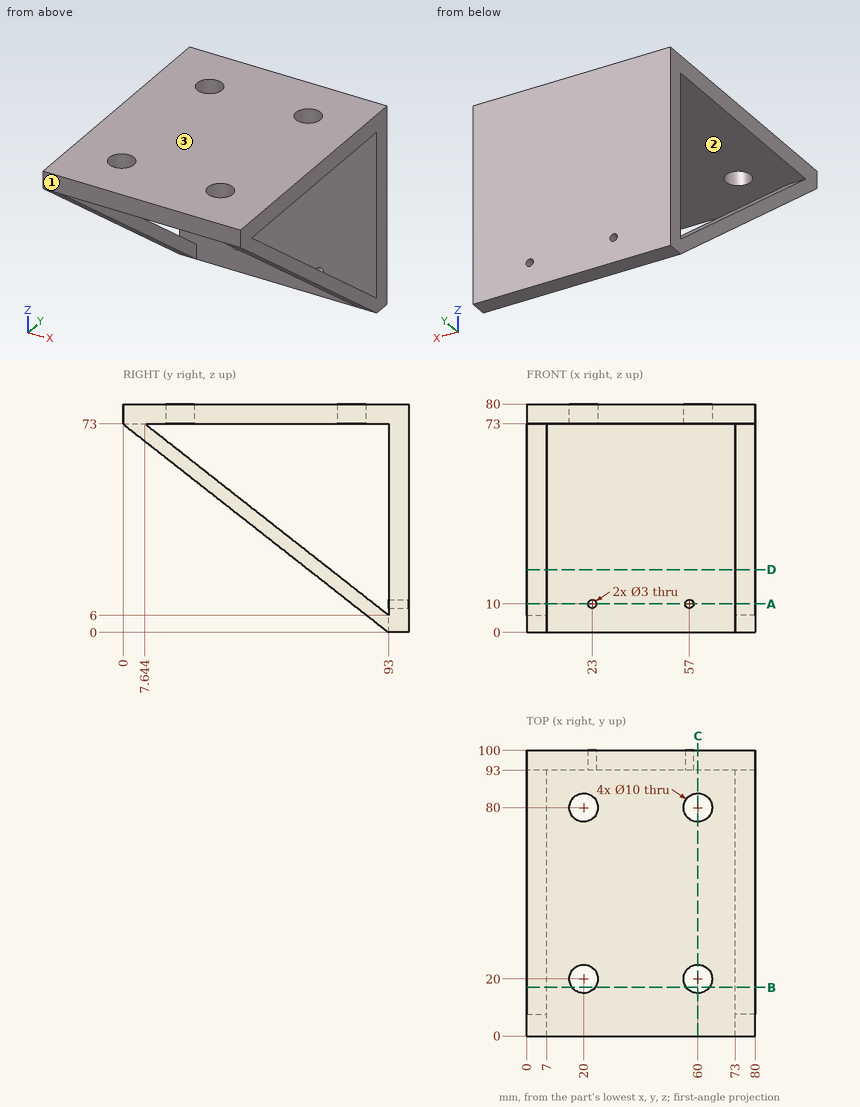
The figure shows three views and two pictorial views of one solid part (mm, origin at its lowest corner). Answer the questions. Round coordinates to 2 decimals unless told otherwise and drop trailing zeros. Write each loop counter-clockwise with the first axis right and the second up, starting at its lowest first coordinate (ties: lowest second). Pieces come first, ordered by that corner, then holes. Notation, with made-up numbers: M 19,49 L 48,49 A20 cw 48,61 Z; hole C -20.75,-35 d5. An arc over 180 degrees is marked long. Write each question's results on one line, items separated by ' | '. Start each with the question number.
(1) Each of these flat-tipped pins is pushed along its axis until it touches: P1, Ø5, axis at x = 14, y = 78.5, coming from the -Z side; P2, Ø3, axis at x = 35, z = 39.5, coming from the -Y side. Where does it stop, or does it pass through?
(2) Find the intervals of material crossed by line 1 (Y direction, x = 20, z = 78); line 2 (X direction, y = 96.25, z = 10); line 3 (Z direction, x = 23, y = 95), in increasing order.
(3) Determine the mould class of the marked faces 1, 2 and 3 for opening direction Z: +Z half, -Z half, draft (parallel to the pull), parting line (faces both ways), or undercut.
(4) The part is cut by section A-A, the plane z = 10. Write down the section's boundary in (x, y), and give its area (3 significant figures).
(5) The part is cut by section C-C, the plane x = 60. Write down the section's boundary in (y, z).
(6) The part is cut by section B-B, the plane y = 17. Write down the section's boundary in (x, z).
(7) The part is cut by section D-D, the plane z = 22. Write down the section's boundary in (x, y).
Worked answers:
1) P1: stops at z = 73 | P2: stops at y = 93
2) line 1: y = 0 to 15, 25 to 75, 85 to 100 | line 2: x = 0 to 21.5, 24.5 to 55.5, 58.5 to 80 | line 3: z = 0 to 8.5, 11.5 to 80
3) face 1: draft | face 2: undercut | face 3: +Z half
4) outline: M 0,80.26 L 7,80.26 L 7,87.9 L 0,87.9 Z; M 0,93 L 21.5,93 L 21.5,100 L 0,100 Z; M 24.5,93 L 55.5,93 L 55.5,100 L 24.5,100 Z; M 58.5,93 L 80,93 L 80,100 L 58.5,100 Z; M 73,80.26 L 80,80.26 L 80,87.9 L 73,87.9 Z | area: 625 mm²
5) outline: M 0,73 L 15,73 L 15,80 L 0,80 Z; M 25,73 L 75,73 L 75,80 L 25,80 Z; M 85,73 L 93,73 L 93,0 L 100,0 L 100,80 L 85,80 Z
6) outline: M 0,59.66 L 7,59.66 L 7,65.66 L 0,65.66 Z; M 0,73 L 16,73 L 16,80 L 0,80 Z; M 24,73 L 56,73 L 56,80 L 24,80 Z; M 64,73 L 80,73 L 80,80 L 64,80 Z; M 73,59.66 L 80,59.66 L 80,65.66 L 73,65.66 Z
7) outline: M 0,64.97 L 7,64.97 L 7,72.62 L 0,72.62 Z; M 0,93 L 80,93 L 80,100 L 0,100 Z; M 73,64.97 L 80,64.97 L 80,72.62 L 73,72.62 Z
